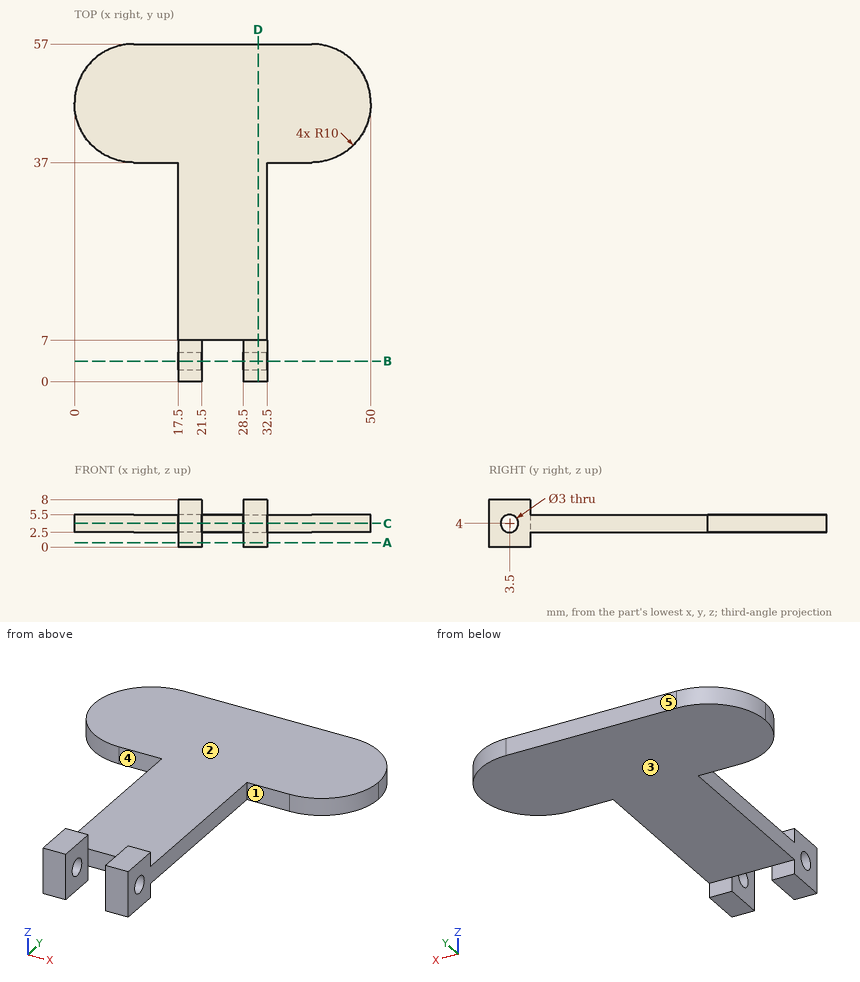
Job drawing, mm, ordinate dimensions from the low corner. One solid piece. A direction names the side the tool comes from. Round coordinates to 2 decimals unless told otherwise and drop trailing zeros. Order: outer loops, then holes, each group sorted by start corner. A loop starts at its lowest first (then second) coordinate and runs counter-clockwise, first axis right, second up. Notation, with made-up numbers: (41, 87.25) -> (91, 87.25) arc R14 ccw to (91, 108.25) -> close; hole circle Ø10 at (57, 81.25). An arc over 180 degrees is marked (long way). Answer in a Markdown table with one row per item.
1) Band-saw the part on A-A on z = 0.75. Give the cut face in (x, y), and give its area (3 significant figures).
Values:
| item | result |
|---|---|
| outline | (17.5, 0) -> (21.5, 0) -> (21.5, 7) -> (17.5, 7) -> close; (28.5, 0) -> (32.5, 0) -> (32.5, 7) -> (28.5, 7) -> close |
| area | 56.0 mm2 |
2) Band-saw the part on D-D on x = 31. Give the cut face in (y, z).
Values:
| item | result |
|---|---|
| outline | (0, 0) -> (7, 0) -> (7, 2.5) -> (57, 2.5) -> (57, 5.5) -> (7, 5.5) -> (7, 8) -> (0, 8) -> close; hole circle Ø3 at (3.5, 4) |
3) Which spindle directions (+Z, -Z, +X, -X, +Y, -Y) get a long thin tool onto all of the face, cutting with end or side? Do the marked faces 1, 2, 3, 4 and 5. Say none if no direction does.
Values:
| item | result |
|---|---|
| face 1 | +Z, -Z, +X, -Y |
| face 2 | +Z, +X, -X, +Y |
| face 3 | -Z, +X, -X, +Y |
| face 4 | +Z, -Z, -X, -Y |
| face 5 | +Z, -Z, +X, -X, +Y |
4) Pin check, flat tips, straight feed: P1, Ø15, axis at x = 22.5, y = 44, coming from the +Z side; P2, Ø0.9, axis at x = 37, z = 4.5, coming from the -Y side; P3, Ø3, axis at x = 23, y = 38, coming from the -Z side. Stop position of each tip, or through.
Values:
| item | result |
|---|---|
| P1 | z = 5.5 |
| P2 | y = 37 |
| P3 | z = 2.5 |
5) Band-saw the part on C-C on z = 4. Give the number of separate pieces and of enclosed holes in the cut face, and give its area (3 significant figures).
Values:
| item | result |
|---|---|
| separate pieces | 3 |
| enclosed holes | 0 |
| area | 1,400 mm2 |
6) Wall check: L1, parallel to Y at x = 18.9, z = 4; L2, parallel to X at y = 5, z = 1.75; L3, parallel to Z at x = 20.15, y = 3.5. Give the ranges that are in metal, low to high.
Values:
| item | result |
|---|---|
| L1 | 0 to 2, 5 to 57 |
| L2 | 17.5 to 21.5, 28.5 to 32.5 |
| L3 | 0 to 2.5, 5.5 to 8 |
7) Band-saw the part on B-B on y = 3.5. Give the cut face in (x, z), and give its area (3 significant figures).
Values:
| item | result |
|---|---|
| outline | (17.5, 0) -> (21.5, 0) -> (21.5, 2.5) -> (17.5, 2.5) -> close; (17.5, 5.5) -> (21.5, 5.5) -> (21.5, 8) -> (17.5, 8) -> close; (28.5, 0) -> (32.5, 0) -> (32.5, 2.5) -> (28.5, 2.5) -> close; (28.5, 5.5) -> (32.5, 5.5) -> (32.5, 8) -> (28.5, 8) -> close |
| area | 40.0 mm2 |
